The model under review builds one solid part; all positions refer to its coordinate system, in mm. Round coordinates to 2 decimals unless told otherwise and drop trailing zeros. Loops run counter-clockwise (first coordinate to the right, second up) from the corner with the lowest first, then second, coordinate; pieces in that order, holes last. Notation, with made-up numbers: M -21.5,71 L 14.5,71 A14 cw 14.5,75 Z; hole C 33,76.25 d6. An arc over 180 degrees is marked long. Answer as a JSON object with one key per item and string values. Group by question number.
Item 1: Insertion check: P1, Ø3, axis at x = 195, z = 2.5, coming from the -Y side; P2, Ø3, axis at y = 204.5, z = 3.5, coming from the +X side. Each pin has a flat end and moves straight along its axis. Give the tip position at first contact, or say it passes through.
Item 2: Consider section B-B (x = 186.5). Give the boundary of the cut face in (y, z).
Item 3: Consider section A-A (z = 3.25). State how many separate pieces and enclosed holes the cut face has, and give its area (3 significant figures).
Item 4: To check wall thickness, follow line 1 (Y direction, x = 222.5, z = 2.5); line 2 (X direction, y = 170.5, z = 1.5); line 3 (X direction, y = -213.5, z = 4.5). State the ranges of each line that lie inside material, in increasing order.
Item 5: Consider section C-C (x = -189). Give the boundary of the cut face in (y, z), and give its area (3 significant figures).
```python
from build123d import *

# Parameters (mm, degrees)
SKETCH1_R           = 2.55
BOSS_EXTRUDE1_DEPTH = 6.35


with BuildPart() as part:
    # Sketch1 → Boss-Extrude1 (new body)
    with BuildSketch(Plane.XY):
        Polygon((12.5, 232.5), (180.5, 232.5), (180.5, 180.5), (232.5, 180.5), (232.5, -180.5), (180.5, -180.5), (180.5, -232.5), (52.5, -232.5), (52.5, -187.5), (-12.5, -187.5), (-12.5, -232.5), (-177.5, -232.5), (-177.5, -182.5), (-232.5, -182.5), (-232.5, 177.5), (-180.5, 177.5), (-180.5, 232.5), (-52.5, 232.5), (-52.5, 187.5), (12.5, 187.5), align=None)
        with Locations((222.5, 170.5)):
            Circle(SKETCH1_R, mode=Mode.SUBTRACT)
        with Locations((170.5, 222.5)):
            Circle(SKETCH1_R, mode=Mode.SUBTRACT)
        with Locations((22.5, 222.5)):
            Circle(SKETCH1_R, mode=Mode.SUBTRACT)
        with Locations((96.5, 222.5)):
            Circle(SKETCH1_R, mode=Mode.SUBTRACT)
        with Locations((-170.5, 222.5)):
            Circle(SKETCH1_R, mode=Mode.SUBTRACT)
        with Locations((-62.5, 222.5)):
            Circle(SKETCH1_R, mode=Mode.SUBTRACT)
        with Locations((-222.5, 167.5)):
            Circle(SKETCH1_R, mode=Mode.SUBTRACT)
        with Locations((222.5, 0)):
            Circle(SKETCH1_R, mode=Mode.SUBTRACT)
        with Locations((222.5, 85.25)):
            Circle(SKETCH1_R, mode=Mode.SUBTRACT)
        with Locations((-222.5, 0)):
            Circle(SKETCH1_R, mode=Mode.SUBTRACT)
        with Locations((-222.5, 83.75)):
            Circle(SKETCH1_R, mode=Mode.SUBTRACT)
        with Locations((222.5, -83.75)):
            Circle(SKETCH1_R, mode=Mode.SUBTRACT)
        with Locations((222.5, -167.5)):
            Circle(SKETCH1_R, mode=Mode.SUBTRACT)
        with Locations((170.5, -222.5)):
            Circle(SKETCH1_R, mode=Mode.SUBTRACT)
        with Locations((62.5, -222.5)):
            Circle(SKETCH1_R, mode=Mode.SUBTRACT)
        with Locations((-22.5, -222.5)):
            Circle(SKETCH1_R, mode=Mode.SUBTRACT)
        with Locations((-96.5, -222.5)):
            Circle(SKETCH1_R, mode=Mode.SUBTRACT)
        with Locations((-170.5, -222.5)):
            Circle(SKETCH1_R, mode=Mode.SUBTRACT)
        with Locations((-222.5, -170.5)):
            Circle(SKETCH1_R, mode=Mode.SUBTRACT)
        with Locations((-222.5, -85.25)):
            Circle(SKETCH1_R, mode=Mode.SUBTRACT)
    extrude(amount=BOSS_EXTRUDE1_DEPTH)


solid = part.part
```
Geometry results:
{
 "1": {"P1": "stops at y = -180.5", "P2": "stops at x = 180.5"},
 "2": {"outline": "M -180.5,0 L 180.5,0 L 180.5,6.35 L -180.5,6.35 Z"},
 "3": {"separate pieces": "1", "enclosed holes": "20", "area": "199,000 mm^2"},
 "4": {"line 1": "y = -180.5 to -170.05, -164.95 to -86.3, -81.2 to -2.55, 2.55 to 82.7, 87.8 to 167.95, 173.05 to 180.5", "line 2": "x = -232.5 to 219.95, 225.05 to 232.5", "line 3": "x = -177.5 to -12.5, 52.5 to 180.5"},
 "5": {"outline": "M -182.5,0 L 177.5,0 L 177.5,6.35 L -182.5,6.35 Z", "area": "2,290 mm^2"}
}
